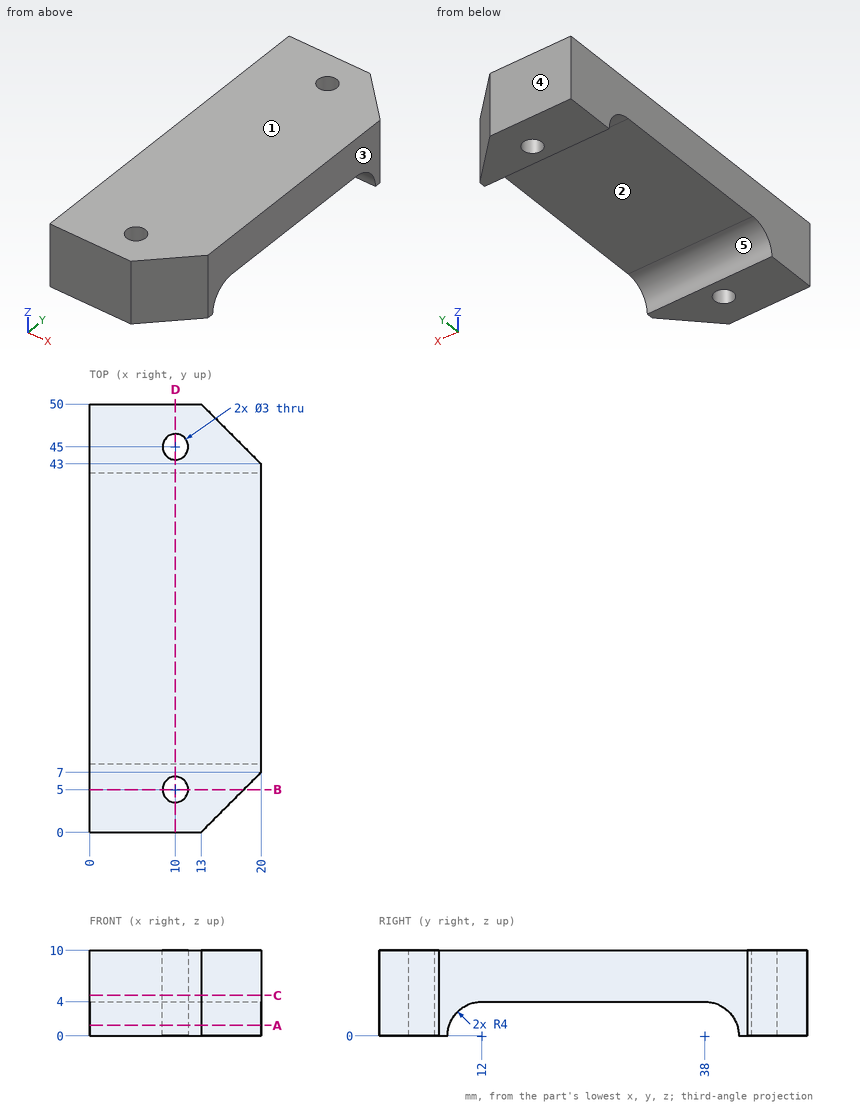
Geometry check sheet. Reference: drawing and pictorial views, mm from the part's lowest x, y, z. A direction names the side the tool comes from. Round coordinates to 2 decimals unless told otherwise and drop trailing zeros. Loops run counter-clockwise (first coordinate to the right, second up) from the corner with the lowest first, then second, coordinate; pieces in that order, holes last. Notation, with made-up numbers: (-28, 60.25) -> (-2, 60.25) arc R9 ccw to (-2, 76.25) -> close; hole circle Ø10 at (41.25, 9.25). An arc over 180 degrees is marked (long way). Answer as a JSON object with one key per item and string values. Group by question number.
Item 1: Cross-section at C-C, the plane z = 4.75. Record the cut outline in (x, y).
Item 2: Set-up check for the marked faces 1 and 2: record each of +Z, -Z, +X, -X, +Y, -Y from which the full face is reachable in a straight line by a thin tool's end or side.
Item 3: Release check for a two-part mould opening along Y. For the marked faces 3, 4 and 5 record: pulls with the +Y half, pulls with the -Y half, needs draft (parallel to the pull), parting line crosses it, or undercut.
Item 4: Cross-section at A-A, the plane z = 1.25. Record the cut outline in (x, y).
Item 5: Depth check by flat-ended pin: pin 1 Ø6 at (x, y) = (14.5, 21.5) entering from -Z. Enter the tip coordinate at first touch or a pass-through.
Item 6: Cross-section at B-B, the plane y = 5. Record the cut outline in (x, z), plus the area to 3 significant figures.
Item 7: Thickness scan on line 1 along Y through (x, z) = (10, 5.5); line 2 along Y through (x, z) = (10, 3); line 3 along Z through (x, y) = (2, 28.5). Record the ranges inside material, lowest first.
Item 8: Cross-section at D-D, the plane x = 10. Record the cut outline in (y, z).
Determined:
{
 "1": {"outline": "(0, 0) -> (13, 0) -> (20, 7) -> (20, 43) -> (13, 50) -> (0, 50) -> close; hole circle Ø3 at (10, 5); hole circle Ø3 at (10, 45)"},
 "2": {"face 1": "+Z, +X, -X, +Y, -Y", "face 2": "-Z, +X, -X"},
 "3": {"face 3": "needs draft", "face 4": "pulls with the +Y half", "face 5": "undercut"},
 "4": {"outline": "(0, 0) -> (13, 0) -> (20, 7) -> (20, 8.2) -> (0, 8.2) -> close; (0, 41.8) -> (20, 41.8) -> (20, 43) -> (13, 50) -> (0, 50) -> close; hole circle Ø3 at (10, 5); hole circle Ø3 at (10, 45)"},
 "5": {"pin 1": "stops at z = 4"},
 "6": {"outline": "(0, 0) -> (8.5, 0) -> (8.5, 10) -> (0, 10) -> close; (11.5, 0) -> (18, 0) -> (18, 10) -> (11.5, 10) -> close", "area": "150 mm²"},
 "7": {"line 1": "y = 0 to 3.5, 6.5 to 43.5, 46.5 to 50", "line 2": "y = 0 to 3.5, 6.5 to 9.35, 40.65 to 43.5, 46.5 to 50", "line 3": "z = 4 to 10"},
 "8": {"outline": "(0, 0) -> (3.5, 0) -> (3.5, 10) -> (0, 10) -> close; (6.5, 0) -> (8, 0) arc R4 cw to (12, 4) -> (38, 4) arc R4 cw to (42, 0) -> (43.5, 0) -> (43.5, 10) -> (6.5, 10) -> close; (46.5, 0) -> (50, 0) -> (50, 10) -> (46.5, 10) -> close"}
}
